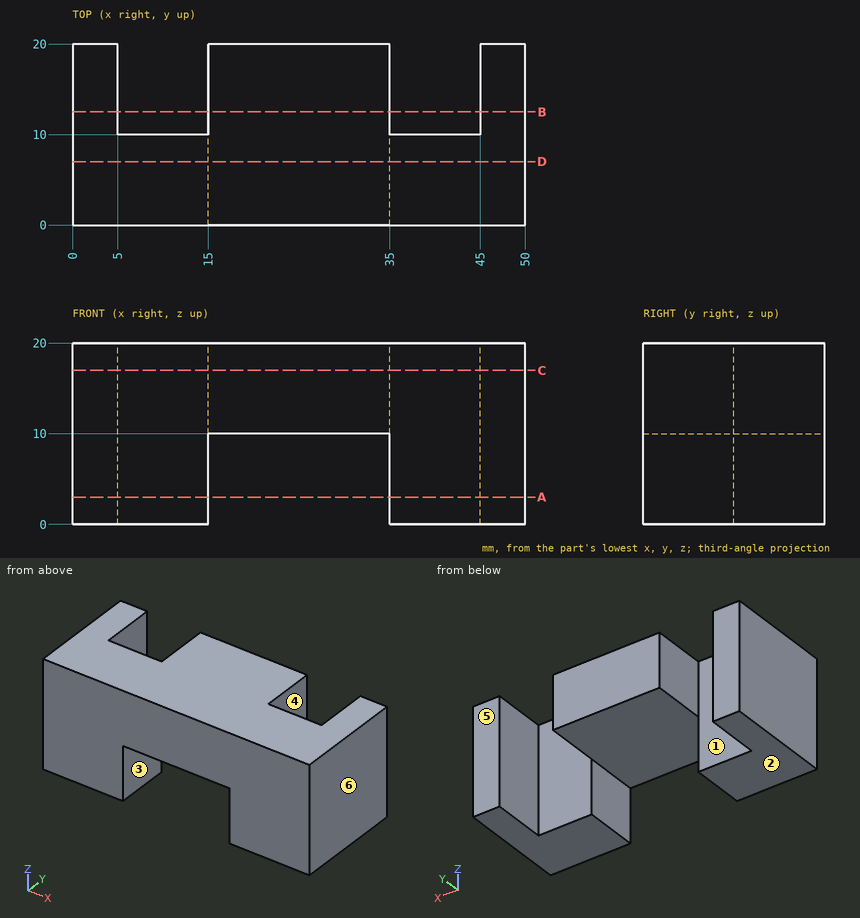
Verification items for this drawing (mm, ordinates from the low corner). A direction names the side the tool comes from. Give positions to 0.01 mm unless a question says otherwise; leave off trailing zeros. Write each loop counter-clockwise with the first axis right and the second up, starting at its lowest first coordinate (ties: lowest second). Pieces come first, ordered by that corner, then holes.
1) Cross-section at D-D (y = 7). Record the boundary of the cut face in (x, z), plus the area to 3 significant figures.
Values follow:
outline: (0, 0) - (15, 0) - (15, 10) - (35, 10) - (35, 0) - (50, 0) - (50, 20) - (0, 20) - close
area: 800 mm2
2) Cross-section at B-B (y = 12.5). Record the boundary of the cut face in (x, z), plus the area to 3 significant figures.
Values follow:
outline: (0, 0) - (5, 0) - (5, 20) - (0, 20) - close; (15, 10) - (35, 10) - (35, 20) - (15, 20) - close; (45, 0) - (50, 0) - (50, 20) - (45, 20) - close
area: 400 mm2
3) Set-up check for the marked faces 1, 2 and 3: record each of +Z, -Z, +X, -X, +Y, -Y from which the full face is reachable in a straight line by a thin tool's end or side.
Values follow:
face 1: +Z, -Z, +Y
face 2: -Z, +X, -X, +Y, -Y
face 3: -Z, +Y, -Y
4) Cross-section at A-A (z = 3). Record the boundary of the cut face in (x, y), plus the area to 3 significant figures.
Values follow:
outline: (0, 0) - (15, 0) - (15, 10) - (5, 10) - (5, 20) - (0, 20) - close; (35, 0) - (50, 0) - (50, 20) - (45, 20) - (45, 10) - (35, 10) - close
area: 400 mm2
5) Release check for a two-part mould opening along X. For the marked faces 4, 5 and 6 record: released by +X, released by -X, zero draft, split by the parting line, or undercut.
Values follow:
face 4: undercut
face 5: zero draft
face 6: released by +X
6) Cross-section at C-C (z = 17). Record the boundary of the cut face in (x, y), plus the area to 3 significant figures.
Values follow:
outline: (0, 0) - (50, 0) - (50, 20) - (45, 20) - (45, 10) - (35, 10) - (35, 20) - (15, 20) - (15, 10) - (5, 10) - (5, 20) - (0, 20) - close
area: 800 mm2
7) Thickness scan on line 1 (X direction, y = 18, z = 13.5); line 2 (X direction, y = 5.5, z = 7.25); line 3 (X direction, y = 16, z = 2.25). Record the ranges inside material, lowest first.
Values follow:
line 1: x = 0 to 5, 15 to 35, 45 to 50
line 2: x = 0 to 15, 35 to 50
line 3: x = 0 to 5, 45 to 50
8) Go/stop test with flat-tipped pins: pin 1 Ø5 at (x, z) = (12.5, 9) entering from +Y; pin 2 Ø10 at (x, y) = (20.5, 12) entering from -Z. Record where each tip stops, or that it passes through.
Values follow:
pin 1: stops at y = 10
pin 2: stops at z = 10
